Verification items for this drawing (mm, ordinates from the low corner). A direction names the side the tool comes from. Round coordinates to 2 decimals unless told otherwise and drop trailing zeros. Loops run counter-clockwise (first coordinate to the right, second up) from the corner with the lowest first, then second, coordinate; pieces in that order, holes last. Notation, with made-up numbers: M 26,88 L 80,88 A11 ccw 80,103 Z; hole C 86.5,68 d7. An arc over 180 degrees is marked long. Use one line per item in the form item = value. Start each with the question number.
1. Set-up check for the marked faces 1, 2 and 3: record each of +Z, -Z, +X, -X, +Y, -Y from which the full face is reachable in a straight line by a thin tool's end or side.
2. Go/stop test with flat-tipped pins: pin 1 (6 mm diameter, centred on x = 28, y = 38, fed in from +Z); pin 2 (16 mm diameter, centred on y = 27.5, z = 6.5, fed in from +X); pin 3 (1 mm diameter, centred on y = 21.5, z = 90, fed in from +X); pin 4 (18 mm diameter, centred on x = 60, y = 55, fed in from +Z). Record where each tip stops, or that it passes through.
3. Cross-section at D-D (z = 59.5). Record the boundary of the cut face in (x, y), then the cut area to 3 significant figures.
4. Draft check along X on the marked faces 4, 5 and 6. Enter one of: pulls with the +X half, pulls with the -X half, needs draft (parallel to the pull), parting line crosses it, or undercut.
5. Material ranges on line 1 (Y direction, x = 60, z = 13); line 2 (X direction, y = 56, z = 80); line 3 (Z direction, x = 99, y = 35.5), recorded low to high.
6. Cross-section at B-B (z = 8). Record the boundary of the cut face in (x, y).
7. Cross-section at A-A (x = 60). Record the boundary of the cut face in (y, z).
8. Cross-section at C-C (y = 55). Record the boundary of the cut face in (x, z).
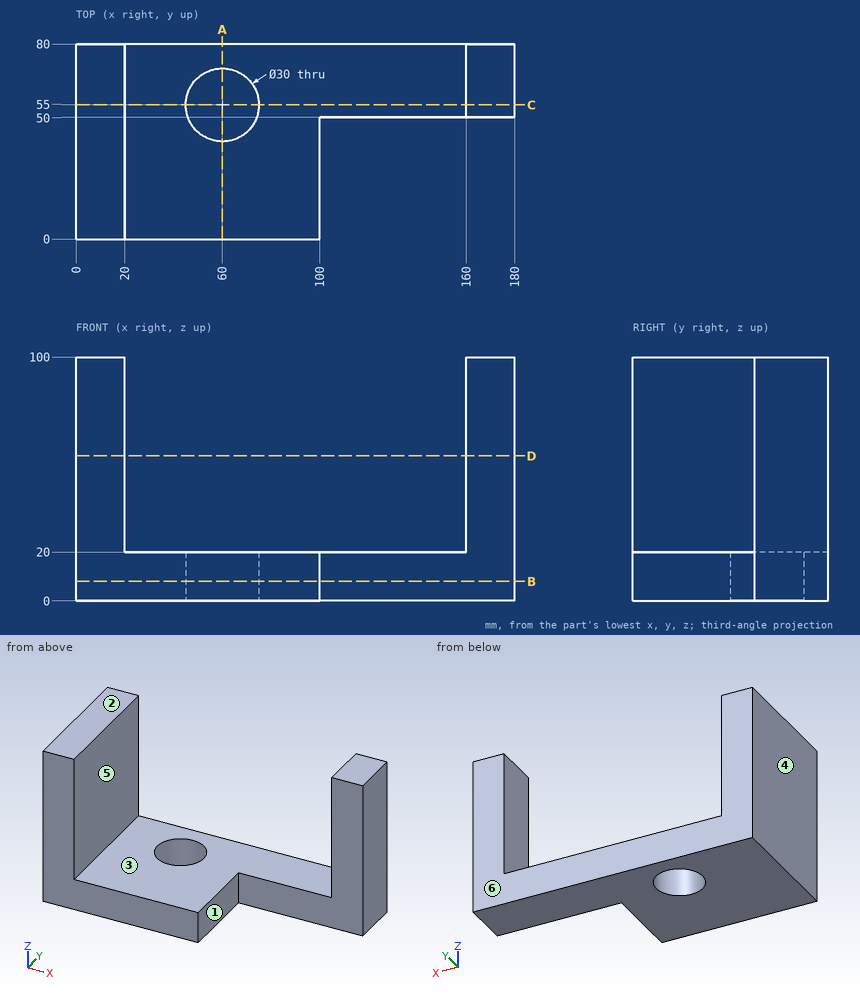
Reported:
q1.face_1 = +Z, -Z, +X, -Y
q1.face_2 = +Z, +X, -X, +Y, -Y
q1.face_3 = +Z, +Y, -Y
q2.pin_1 = 20
q2.pin_2 = 100
q2.pin_3 = 20
q2.pin_4 = through
q3.outline = M 0,0 L 20,0 L 20,80 L 0,80 Z; M 160,50 L 180,50 L 180,80 L 160,80 Z
q3.area = 2,200 mm²
q4.face_4 = pulls with the -X half
q4.face_5 = undercut
q4.face_6 = needs draft
q5.line_1 = 0 to 40, 70 to 80
q5.line_2 = 0 to 20, 160 to 180
q5.line_3 = 0 to 20
q6.outline = M 0,0 L 100,0 L 100,50 L 180,50 L 180,80 L 0,80 Z; hole C 60,55 d30
q7.outline = M 0,0 L 40,0 L 40,20 L 0,20 Z; M 70,0 L 80,0 L 80,20 L 70,20 Z
q8.outline = M 0,0 L 45,0 L 45,20 L 20,20 L 20,100 L 0,100 Z; M 75,0 L 180,0 L 180,100 L 160,100 L 160,20 L 75,20 Z
